Part print with two shaded views. Sizes in mm from the minimum x, y, z corner. Give positions to 0.01 mm unless a question says otherwise; leave off trailing zeros. Write each loop counter-clockwise with the first axis right and the second up, starting at its lowest first coordinate (ties: lowest second). Pieces come first, ordered by that corner, then holes. Notation, with made-up numbers: (80.25, 20) -> (130.25, 20) arc R13 cw to (130.25, 39) -> close; hole circle Ø5 at (-34, -34.75). An arc over 180 degrees is marked (long way). Answer as a JSON object with one key per item and string values.
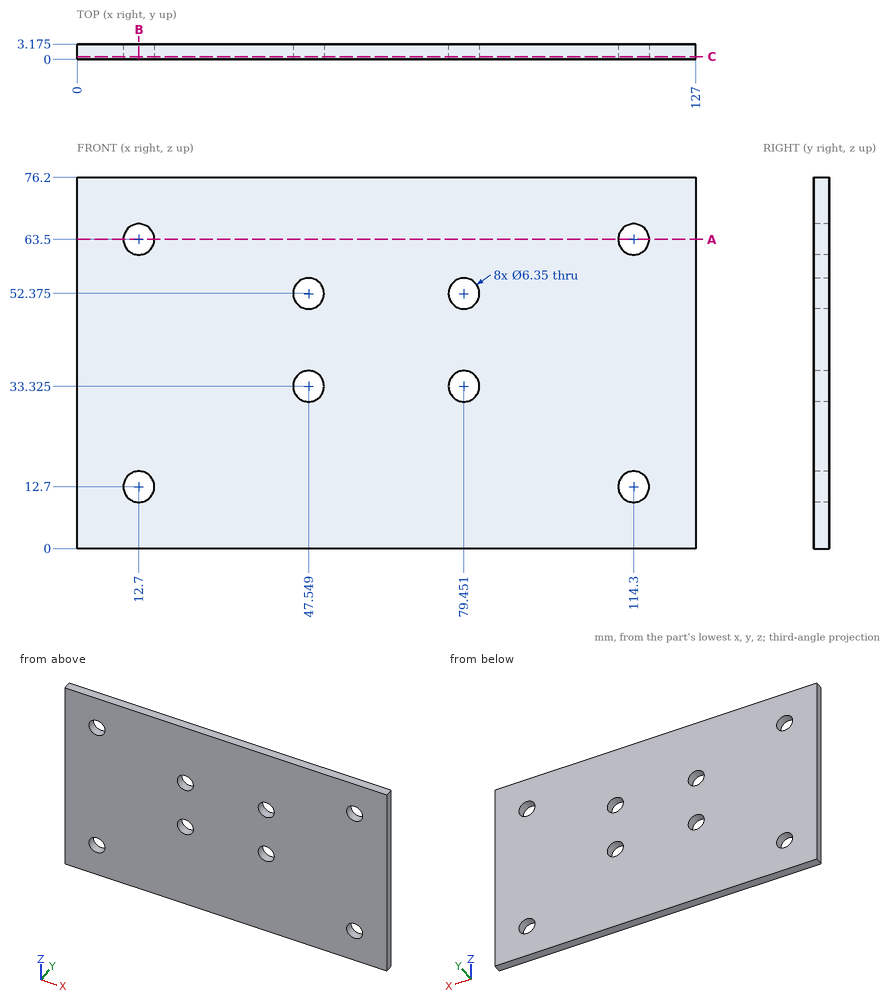
1) Slice it at C-C (y = 0.6). State how many separate pieces and enclosed holes the cut face has, then the cut area to 3 significant figures.
Model answer:
{"separate pieces": "1", "enclosed holes": "8", "area": "9,420 mm2"}
2) Pin check, flat tips, straight feed: pin 1 (5.5 mm diameter, centred on x = 114.3, z = 12.7, fed in from +Y); pin 2 (3 mm diameter, centred on x = 36, z = 46.5, fed in from -Y). Stop position of each tip, or through.
Model answer:
{"pin 1": "passes through", "pin 2": "stops at y = 0"}
3) Wall check: probe 1 along X at (y, z) = (1.9, 63.5) (3 decimals); probe 2 along Z at (x, y) = (79.5, 2.75); probe 3 along X at (y, z) = (2.2, 61). Give the ranges that are in metal, low to high.
Model answer:
{"probe 1": "x = 0 to 9.525, 15.875 to 111.125, 117.475 to 127", "probe 2": "z = 0 to 30.15, 36.5 to 49.2, 55.55 to 76.2", "probe 3": "x = 0 to 10.74, 14.66 to 112.34, 116.26 to 127"}
4) Slice it at A-A (z = 63.5). List the corners of the cut face in (x, y) (3 decimals).
Model answer:
{"outline": "(0, 0) -> (9.525, 0) -> (9.525, 3.175) -> (0, 3.175) -> close; (15.875, 0) -> (111.125, 0) -> (111.125, 3.175) -> (15.875, 3.175) -> close; (117.475, 0) -> (127, 0) -> (127, 3.175) -> (117.475, 3.175) -> close"}
5) Slice it at B-B (x = 12.7). List the corners of the cut face in (y, z) (3 decimals).
Model answer:
{"outline": "(0, 0) -> (3.175, 0) -> (3.175, 9.525) -> (0, 9.525) -> close; (0, 15.875) -> (3.175, 15.875) -> (3.175, 60.325) -> (0, 60.325) -> close; (0, 66.675) -> (3.175, 66.675) -> (3.175, 76.2) -> (0, 76.2) -> close"}
